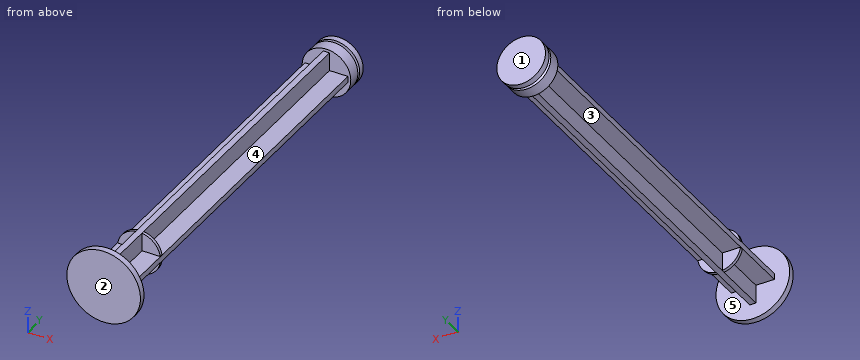
```python
from build123d import *

# Parameters (mm, degrees)
SKETCH1_R      = 6
EXTRUDE1_DEPTH = 1
EXTRUDE2_DEPTH = 62
SKETCH5_R      = 3.5
EXTRUDE4_DEPTH = 0.5
SKETCH6_R      = 0.53375681
EXTRUDE5_DEPTH = 1.5
SKETCH7_R      = 3.962531225
EXTRUDE6_DEPTH = 2.5
CHAMFER1_SIZE  = 0.5
SKETCH8_R      = 3.96497508
EXTRUDE7_DEPTH = 1


with BuildPart() as part:
    # Sketch1 → Extrude1 (new body)
    with BuildSketch(Plane(origin=(0, 0, 0), x_dir=(1, 0, 0), z_dir=(0, 1, 0))):
        with Locations(Location((0, 0, 0), (0, 0, 270))):
            Circle(SKETCH1_R)
    extrude(amount=EXTRUDE1_DEPTH)

    # Sketch2 → Extrude2 (add)
    with BuildSketch(Plane(origin=(0, 1, 0), x_dir=(-1, 0, 0), z_dir=(0, 1, 0))):
        Polygon((0.5, 0.5), (0.5, 3.5), (-0.5, 3.5), (-0.5, 0.5), (-3.5, 0.5), (-3.5, -0.5), (-0.5, -0.5), (-0.5, -3.5), (0.5, -3.5), (0.5, -0.5), (3.5, -0.5), (3.5, 0.5), align=None)
    extrude(amount=EXTRUDE2_DEPTH)

    # Sketch5 → Extrude4 (add)
    with BuildSketch(Plane(origin=(0, 10, 0), x_dir=(-1, 0, 0), z_dir=(0, 1, 0))):
        Circle(SKETCH5_R)
    extrude(amount=EXTRUDE4_DEPTH)

    # Sketch6 → Extrude5 (add)
    with BuildSketch(Plane(origin=(0, 63, 0), x_dir=(-1, 0, 0), z_dir=(0, 1, 0))):
        with Locations(Location((0, 0, 0), (0, 0, 270))):
            Circle(SKETCH6_R)
    extrude(amount=EXTRUDE5_DEPTH)

    # Sketch7 → Extrude6 (add)
    with BuildSketch(Plane(origin=(0, 63, 0), x_dir=(-1, 0, 0), z_dir=(0, 1, 0))):
        with Locations(Location((0, 0, 0), (0, 0, 90))):
            Circle(SKETCH7_R)
    extrude(amount=EXTRUDE6_DEPTH)

    # Chamfer1
    chamfer1_edges = [part.edges().sort_by_distance(p)[0] for p in [
        (0, 65.5, -3.962531225),
    ]]
    chamfer(chamfer1_edges, length=CHAMFER1_SIZE)

    # Sketch8 → Extrude7 (add)
    with BuildSketch(Plane(origin=(0, 65.5, 0), x_dir=(-1, 0, 0), z_dir=(0, 1, 0))):
        with Locations(Location((0, 0, 0), (0, 0, 90))):
            Circle(SKETCH8_R)
    extrude(amount=EXTRUDE7_DEPTH)


solid = part.part
```
Check sheet for the modelled part. Datum: model origin and axes. Units: mm. Face numbers are marked on the shaded views. A direction names the side the tool comes from. Give positions to 0.01 mm unless a question says otherwise; leave off trailing zeros. Order: outer loops, then holes, each group sorted by start corner. A loop starts at its lowest first (then second) coordinate and runs counter-clockwise, first axis right, second up. Notation, with made-up numbers: M -10,29 L 2,29 A21 cw 2,43 Z; hole C -24,-29.5 d2. An arc over 180 degrees is marked long. Answer in a Markdown table with one row per item. Add a question column.
Q1. Thickness scan on L1, parallel to Y at x = -0.5, z = -3.75; L2, parallel to Z at x = -2.5, y = 36. Record the ranges inside material, lowest first.
Q2. Sectioned sample at A-A, the plane y = 8. Record the boundary of the cut face in (x, z).
Q3. Sectioned sample at C-C, the plane z = -5. Record the boundary of the cut face in (x, y), and give its area (3 significant figures).
Q4. Gauge pin test, flat ends, axial feed: pin 1 Ø3.5 at (y, z) = (24.5, -2.5) entering from +X; pin 2 Ø1.5 at (x, y) = (-3.5, 16.5) entering from +Z; pin 3 Ø6 at (y, z) = (50.5, -0.5) entering from +X. Record the tip position at first contact, or that the pin passes through.
Q5. Sectioned sample at B-B, the plane z = 4.75. Record the boundary of the cut face in (x, y), and give its area (3 significant figures).
Q6. Release check for a two-part mould opening along Y. For the marked faces 1, 2 and 3 record: released by +Y, released by -Y, zero draft, split by the parting line, or undercut.
Q7. Access from +Z, -Z, +X, -X, +Y, -Y to the whole of each face (thin tool, end or side, straight path). Record for the marked faces 4 and 5.
Verdict:
| question | item | result |
|---|---|---|
| 1 | L1 | 0 to 1, 63 to 65.18, 65.5 to 66.5 |
| 1 | L2 | -0.5 to 0.5 |
| 2 | outline | M -3.5,-0.5 L -0.5,-0.5 L -0.5,-3.5 L 0.5,-3.5 L 0.5,-0.5 L 3.5,-0.5 L 3.5,0.5 L 0.5,0.5 L 0.5,3.5 L -0.5,3.5 L -0.5,0.5 L -3.5,0.5 Z |
| 3 | outline | M -3.32,0 L 3.32,0 L 3.32,1 L -3.32,1 Z |
| 3 | area | 6.63 mm² |
| 4 | pin 1 | x = 0.5 |
| 4 | pin 2 | z = 0.5 |
| 4 | pin 3 | x = 3.5 |
| 5 | outline | M -3.67,0 L 3.67,0 L 3.67,1 L -3.67,1 Z |
| 5 | area | 7.33 mm² |
| 6 | face 1 | released by +Y |
| 6 | face 2 | released by -Y |
| 6 | face 3 | undercut |
| 7 | face 4 | +Z, +X |
| 7 | face 5 | none |
